```python
from build123d import *

# Parameters (mm, degrees)
SKETCH001_W         = 10
SKETCH001_H         = 15
PAD001_DEPTH        = 21
FILLET001_R         = 7.499
SKETCH005_W         = 10
SKETCH005_H         = 15
PAD002_DEPTH        = 21
FILLET002_R         = 7.499
PAD_DEPTH           = 4
FILLET_R            = 1
SKETCH008_W         = 6
SKETCH008_H         = 4
PAD003_DEPTH        = 8
SKETCH009_W         = 6
SKETCH009_H         = 4
PAD004_DEPTH        = 8
SKETCH010_W         = 6
SKETCH010_H         = 4
PAD005_DEPTH        = 8
SKETCH011_W         = 6
SKETCH011_H         = 4
PAD006_DEPTH        = 8
FILLET003_R         = 1
HOLE001_D           = 3
HOLE001_DEPTH       = 100
HOLE001_CBORE_D     = 6
HOLE001_CBORE_DEPTH = 3
SKETCH013_W         = 3
SKETCH013_H         = 2
POCKET_DEPTH        = 15
SKETCH014_W         = 3
SKETCH014_H         = 2
POCKET001_DEPTH     = 15


with BuildPart() as left_hinge:
    # Sketch001 → Pad001 (new body)
    with BuildSketch(Plane.XZ):
        with Locations((-9.75, 0)):
            Rectangle(SKETCH001_W, SKETCH001_H)
    extrude(amount=PAD001_DEPTH)

    # Fillet001
    fillet001_edges = [left_hinge.edges().sort_by_distance(p)[0] for p in [
        (-9.75, -21, -7.5),
        (-9.75, -21, 7.5),
    ]]
    fillet(fillet001_edges, radius=FILLET001_R)


with BuildPart() as body002:
    # Sketch005 → Pad002 (new body)
    with BuildSketch(Plane.XZ):
        with Locations((9.75, 0)):
            Rectangle(SKETCH005_W, SKETCH005_H)
    extrude(amount=PAD002_DEPTH)

    # Fillet002
    fillet002_edges = [body002.edges().sort_by_distance(p)[0] for p in [
        (9.75, -21, -7.5),
        (9.75, -21, 7.5),
    ]]
    fillet(fillet002_edges, radius=FILLET002_R)


with BuildPart() as base:
    # Sketch → Pad (new body)
    with BuildSketch(Plane.XZ):
        Polygon((-35, 10), (-1, 10), (0, 8.267949), (1, 10), (35, 10), (35, 1), (33.267949, 0), (35, -1), (35, -10), (1, -10), (0, -8.267949), (-1, -10), (-35, -10), (-35, -1), (-33.267949, 0), (-35, 1), align=None)
        with BuildLine():
            ThreePointArc((-28, 1.5), (-29.5, 0), (-28, -1.5))
            Line((-28, -1.5), (-22, -1.5))
            ThreePointArc((-22, -1.5), (-20.5, 0), (-22, 1.5))
            Line((-28, 1.5), (-22, 1.5))
        make_face(mode=Mode.SUBTRACT)
        with BuildLine():
            ThreePointArc((22, 1.5), (20.5, 0), (22, -1.5))
            Line((22, -1.5), (28, -1.5))
            ThreePointArc((28, -1.5), (29.5, 0), (28, 1.5))
            Line((22, 1.5), (28, 1.5))
        make_face(mode=Mode.SUBTRACT)
    extrude(amount=PAD_DEPTH)

    # Fillet
    fillet_edges = [base.edges().sort_by_distance(p)[0] for p in [
        (-18, -4, -10),
        (18, -4, -10),
        (35, -4, -5.5),
        (35, -4, 5.5),
        (18, -4, 10),
        (-18, -4, 10),
        (-35, -4, 5.5),
        (-35, -4, -5.5),
    ]]
    fillet(fillet_edges, radius=FILLET_R)

    # Boolean: union Left hinge
    add(left_hinge.part)

    # Boolean001: union Body002
    add(body002.part)

    # Sketch008 → Pad003 (join)
    with BuildSketch(Plane.XZ):
        with Locations((-31, 7)):
            Rectangle(SKETCH008_W, SKETCH008_H)
    extrude(amount=PAD003_DEPTH)

    # Sketch009 → Pad004 (join)
    with BuildSketch(Plane.XZ):
        with Locations((31, 7)):
            Rectangle(SKETCH009_W, SKETCH009_H)
    extrude(amount=PAD004_DEPTH)

    # Sketch010 → Pad005 (join)
    with BuildSketch(Plane.XZ):
        with Locations((-31, -7)):
            Rectangle(SKETCH010_W, SKETCH010_H)
    extrude(amount=PAD005_DEPTH)

    # Sketch011 → Pad006 (join)
    with BuildSketch(Plane.XZ):
        with Locations((31, -7)):
            Rectangle(SKETCH011_W, SKETCH011_H)
    extrude(amount=PAD006_DEPTH)

    # Fillet003
    fillet003_edges = [base.edges().sort_by_distance(p)[0] for p in [
        (-34, -8, 7),
        (-31, -8, 5),
        (-28, -8, 7),
        (-31, -8, 9),
        (-34, -8, -7),
        (-31, -8, -9),
        (-28, -8, -7),
        (-31, -8, -5),
        (28, -8, -7),
        (31, -8, -9),
        (34, -8, -7),
        (31, -8, -5),
        (28, -8, 7),
        (31, -8, 5),
        (34, -8, 7),
        (31, -8, 9),
    ]]
    fillet(fillet003_edges, radius=FILLET003_R)

    # Hole001
    with Locations(Plane.YZ.offset(14.75)):
        with Locations((-13.5, 0)):
            CounterBoreHole(HOLE001_D / 2, HOLE001_CBORE_D / 2, HOLE001_CBORE_DEPTH, depth=HOLE001_DEPTH)

    # Sketch013 → Pocket (cut, symmetric)
    with BuildSketch(Plane.XY):
        with Locations((-31, -5)):
            Rectangle(SKETCH013_W, SKETCH013_H)
    extrude(amount=POCKET_DEPTH, both=True, mode=Mode.SUBTRACT)

    # Sketch014 → Pocket001 (cut, symmetric)
    with BuildSketch(Plane.XY):
        with Locations((31.120665, -5)):
            Rectangle(SKETCH014_W, SKETCH014_H)
    extrude(amount=POCKET001_DEPTH, both=True, mode=Mode.SUBTRACT)


solid = base.part
```
Can you work these out from the model? Positions are in its coordinate system, mm. A direction names the side the tool comes from. Round coordinates to 2 decimals unless told otherwise and drop trailing zeros. Loops run counter-clockwise (first coordinate to the right, second up) from the corner with the lowest first, then second, coordinate; pieces in that order, holes last. Notation, with made-up numbers: (15, 6) -> (37, 6) arc R26 cw to (37, 24) -> close; hole circle Ø9 at (83, 43.5). An arc over 180 degrees is marked (long way). One line per item, written item: value. Start each with the question number.
1. If I drill on probe 1 along X at (y, z) = (-4.5, -8.75); probe 2 along Z at (x, y) = (-7.25, -13.5); probe 3 along X at (y, z) = (-7.5, 4.25), over which ranges is the centre line in solid material (lowest first)?
2. If we section it at B-B, the plane x = -2: Write out the boundary of the cut face in (y, z), then the cut area to 3 significant figures.
3. If we section it at A-A, the plane y = -17.25: Write out the boundary of the cut face in (x, z).
4. If we mould it in two halves opening along Y, with no side actions, what happens to faces 4 (the flat face through (31, -8, 7)), 5 (the flat face through (-31, -6, -7)), 6 (the cylindrical face through (20.5, -2, 0))? For each: pulls with the +Y half, pulls with the -Y half, needs draft (parallel to the pull), parting line crosses it, or undercut.
5. For faces 1 (the flat face through (-31.04, -6.15, 9)), 2 (the flat face through (-34, -5, 7)), 3 (the flat face through (10, -9, -7.5)), which set-ups out of +Z, -Z, +X, -X, +Y, -Y let a thin tool reach every point of the face, with its end or its side?
6. If we section it at C-C, the plane z = -6.75: Give the number of separate pieces and of enclosed holes in the cut face, then the cut area to 3 significant figures.
7. For pin 1 (3.5 mm diameter, centred on x = 31.5, y = -5.5, fed in from +Z); pin 2 (2 mm diameter, centred on x = 12, y = -9, fed in from +Z); pin 3 (1.5 mm diameter, centred on y = -6, z = -6.5, fed in from +X); pin 4 (10 mm diameter, centred on x = 3, z = 5, fed in from +Y), each with a flat end and sliding along its axis, tell me the tip position at first contact or that it passes through.
Calculated:
1. probe 1: x = -34 to -32.5, -29.5 to -28, 28 to 29.62, 32.62 to 34
1. probe 2: z = -7.5 to -1.5, 1.5 to 7.5
1. probe 3: x = -14.75 to -4.75, 4.75 to 14.75
2. outline: (-4, -9) arc R1 ccw to (-3, -10) -> (0, -10) -> (0, 10) -> (-3, 10) arc R1 ccw to (-4, 9) -> close
2. area: 79.6 mm²
3. outline: (-14.75, -6.5) -> (-4.75, -6.5) -> (-4.75, 6.5) -> (-14.75, 6.5) -> close; (4.75, -6.5) -> (14.75, -6.5) -> (14.75, 6.5) -> (4.75, 6.5) -> close
4. face 4: pulls with the -Y half
4. face 5: undercut
4. face 6: needs draft
5. face 1: +Z, +X, -X, -Y
5. face 2: +Z, -Z, -X, -Y
5. face 3: -Z, -Y
6. separate pieces: 1
6. enclosed holes: 2
6. area: 570 mm²
7. pin 1: stops at z = 9.66
7. pin 2: stops at z = 7.5
7. pin 3: stops at x = 34
7. pin 4: stops at y = 0
